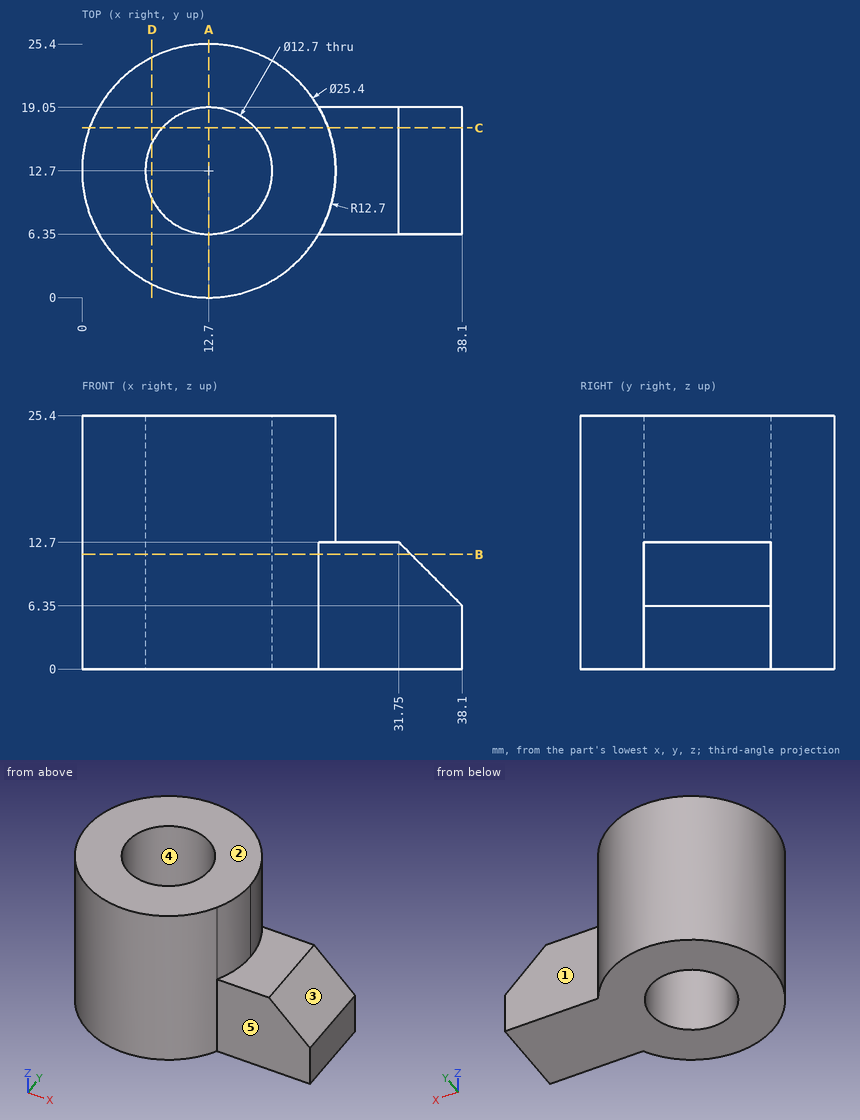
Can you work these out from the drawing? Everything is in mm from the part's minimum corner. A direction names the side the tool comes from. Coordinates: 2 decimals unless noted, no trailing zeros. Loops run counter-clockwise (first coordinate to the right, second up) from the corner with the lowest first, then second, coordinate; pieces in that order, holes last. Notation, with made-up numbers: (30, 52) - (82, 52) arc R17 cw to (82, 67) - close; hole circle Ø11 at (39, 21). An arc over 180 degrees is marked (long way). Put each result on its own line as item: value. Start each with the question number.
Item 1: Suppose I cut it at D-D (x = 7). Please give me the cut outline in (y, z).
Item 2: Suppose I cut it at B-B (z = 11.5). Please give me the cut outline in (x, y), and give its area (3 significant figures).
Item 3: If I drill on line 1 along X through (y, z) = (13, 21.5); line 2 along Y through (x, z) = (31.5, 6); line 3 along X through (y, z) = (17.5, 7), over which ranges is the centre line in solid material (lowest first)?
Item 4: Suppose I cut it at A-A (x = 12.7). Please give me the cut outline in (y, z).
Item 5: For pin 1 (3 mm diameter, centred on y = 10, z = 17, fed in from +X); pin 2 (10 mm diameter, centred on y = 20.5, z = 21.5, fed in from +X); pin 3 (10 mm diameter, centred on x = 31.5, z = 5.5, fed in from +Y), each with a flat end and sliding along its axis, tell me the tip position at first contact or that it passes through.
Item 6: Suppose I cut it at C-C (y = 17). Please give me the cut outline in (x, z), and give its area (3 significant figures).
Item 7: If we mould it in two halves opening along Y, with no side actions, what happens to the marked faces 3, 4 and 5? For each: +Y half, -Y half, draft (parallel to the pull), parting line (faces both ways), or undercut.
Item 8: Which directions (+Z, -Z, +X, -X, +Y, -Y) give clear straight access to the entire face, cutting with the end or side of a thin tool? Please do the marked faces 1 and 2.
Here are the results:
1. outline: (1.35, 0) - (9.9, 0) - (9.9, 25.4) - (1.35, 25.4) - close; (15.5, 0) - (24.05, 0) - (24.05, 25.4) - (15.5, 25.4) - close
2. outline: (23.7, 6.35) - (32.95, 6.35) - (32.95, 19.05) - (23.7, 19.05) arc R12.7 ccw (long way) to start; hole circle Ø12.7 at (12.7, 12.7)
2. area: 483 mm²
3. line 1: 0 to 6.36, 19.04 to 25.4
3. line 2: 6.35 to 19.05
3. line 3: 0.94 to 8.54, 16.86 to 37.45
4. outline: (0, 0) - (6.35, 0) - (6.35, 25.4) - (0, 25.4) - close; (19.05, 0) - (25.4, 0) - (25.4, 25.4) - (19.05, 25.4) - close
5. pin 1: x = 25.34
5. pin 2: x = 25.09
5. pin 3: y = 19.05
6. outline: (0.75, 0) - (8.03, 0) - (8.03, 25.4) - (0.75, 25.4) - close; (17.37, 0) - (38.1, 0) - (38.1, 6.35) - (31.75, 12.7) - (24.65, 12.7) - (24.65, 25.4) - (17.37, 25.4) - close
6. area: 520 mm²
7. face 3: draft
7. face 4: undercut
7. face 5: -Y half
8. face 1: +Z, -Z, +X, +Y
8. face 2: +Z, +X, -X, +Y, -Y
